Read the model definition and answer for the solid it produces. Units are mm, in the model's axes. A direction names the side the tool comes from. Round coordinates to 2 decimals unless told otherwise and drop trailing zeros. Order: outer loops, then holes, each group sorted by start corner. A loop starts at its lowest first (then second) coordinate and runs counter-clockwise, first axis right, second up. Notation, with made-up numbers: (17.25, 52.25) -> (74.25, 52.25) arc R30 ccw to (74.25, 83.25) -> close; hole circle Ø3 at (50, 9.25). An arc over 180 degrees is marked (long way). Answer as a JSON object with one key per item and string values. Group by question number.
Item 1: For faces 4 (the flat face through (15, 2.4, -2.4)), 5 (the flat face through (93, -12.457, 0)), 6 (the flat face through (52.7, 14.15, -0.07)), determine the directions among +Z, -Z, +X, -X, +Y, -Y from which every point of the face is accessible in a straight line to the end or side of a thin tool.
Item 2: Consider probe 1 along X at (y, z) = (8.5, -3); probe 2 along X at (y, z) = (-10, 5); probe 3 along Z at (x, y) = (85.5, -1). Determine where each line is inside the solid, lowest interval first. Write a range as from..to.
Item 3: The mould has two halves that part along Z. Classify faces 1 (the flat face through (18, 9, 0)), 2 (the cylindrical face through (20.679, 10.657, 9.518)), 3 (the cylindrical face through (94.47, -0.05, -1.25)): pulls with the +Z half, pulls with the -Z half, needs draft (parallel to the pull), parting line crosses it, or undercut.
Item 4: Given P1, Ø0.8, axis at y = 0.5, z = 0, coming from the +X side; P2, Ø4, axis at x = 16, y = 3.5, coming from the -Z side; P3, Ø1.5, axis at x = 93, z = 0, coming from the -Y side, each flat-ended and moving along its own axis, determine where each tip first touches the part or whether it passes through.
Item 5: Section B-B, the plane x = 43 is taken. Write down the section's boundary in (y, z), plus the area to 3 significant figures.
from build123d import *

# Parameters (mm, degrees)
SKETCH_2_OUTSIDE_W       = 55.172
SKETCH_2_OUTSIDE_H       = 55.172
SKETCH_2_OUTSIDE_W_2     = 20
SKETCH_2_OUTSIDE_H_2     = 18
CUT_EXTRUDE_1_DEPTH      = 3
CHAMFER_1_SIZE           = 1
SKETCH_3_R               = 1.5
CUT_EXTRUDE_3_DEPTH      = 3
PATTERN_CIRCULAR_2_COUNT = 4
EXTRUDE_2_DEPTH          = 6
PATTERN_CIRCULAR_3_COUNT = 2


with BuildPart() as part:
    # ｽｹｯﾁ1 → 回転2 (revolve)
    with BuildSketch(Plane(origin=(0, 0, 0), x_dir=(1, 0, 0), z_dir=(0, 1, 0)), mode=Mode.PRIVATE) as revolve_2_sk:
        Polygon((0, 0), (0, 3), (15, 3), (15, 5.5), (15.8, 5.5), (15.8, 7), (16.2, 7), (16.2, 10), (19.2, 10), (19.2, 16), (52.7, 16), (52.7, 14), (90.2, 14), (90.2, 5), (93.2, 5), (93.2, 1.25), (95.7, 1.25), (95.7, 0), align=None)
    revolve(revolve_2_sk.sketch.rotate(Axis((0, 0, 0), (1, 0, 0)), 180), axis=Axis((0, 0, 0), (1, 0, 0)))

    # ｽｹｯﾁ2 outside → ｶｯﾄ - 押し出し1 (cut)
    with BuildSketch(Plane.ZY.offset(-16.2)):
        Rectangle(SKETCH_2_OUTSIDE_W, SKETCH_2_OUTSIDE_H)
        Rectangle(SKETCH_2_OUTSIDE_W_2, SKETCH_2_OUTSIDE_H_2, mode=Mode.SUBTRACT)
    extrude(amount=-CUT_EXTRUDE_1_DEPTH, mode=Mode.SUBTRACT)

    # 面取り1
    chamfer_1_edges = [part.edges().sort_by_distance(p)[0] for p in [
        (19.2, 0, -16),
    ]]
    chamfer(chamfer_1_edges, length=CHAMFER_1_SIZE)

    # ｽｹｯﾁ3 → ｶｯﾄ - 押し出し3 (cut)
    with BuildSketch(Plane.ZY.offset(-19.2)):
        with Locations((-9.192388155, -9.192388155)):
            Circle(SKETCH_3_R)
    cut_extrude_3 = extrude(amount=-CUT_EXTRUDE_3_DEPTH, mode=Mode.SUBTRACT)

    # 円形ﾊﾟﾀｰﾝ2: ｶｯﾄ - 押し出し3 ×4 about axis
    pattern_circular_2_axis = Axis((0, 0, 0), (1, 0, 0))
    for i in range(1, PATTERN_CIRCULAR_2_COUNT):
        add(cut_extrude_3.rotate(pattern_circular_2_axis, i * 360 / PATTERN_CIRCULAR_2_COUNT), mode=Mode.SUBTRACT)

    # ｽｹｯﾁ4 → ﾎﾞｽ - 押し出し2 (add)
    with BuildSketch(Plane(origin=(90.2, 0, 0), x_dir=(0, 0, -1), z_dir=(1, 0, 0))):
        Polygon((0, 12.956973635), (2.5, 12.956973635), (2.5, 12.456973635), (-2.5, 12.456973635), (-2.5, 12.956973635), align=None)
    extrude_2 = extrude(amount=EXTRUDE_2_DEPTH)

    # 円形ﾊﾟﾀｰﾝ3: ﾎﾞｽ - 押し出し2 ×2 about axis
    pattern_circular_3_axis = Axis((0, 0, 0), (1, 0, 0))
    for i in range(1, PATTERN_CIRCULAR_3_COUNT):
        add(extrude_2.rotate(pattern_circular_3_axis, i * 360 / PATTERN_CIRCULAR_3_COUNT))


solid = part.part
Values found:
{
 "1": {"face 4": "-X", "face 5": "+Z, -Z, +X", "face 6": "+X"},
 "2": {"probe 1": "16.2..90.2", "probe 2": "19.2..90.2", "probe 3": "-13.96..13.96"},
 "3": {"face 1": "needs draft", "face 2": "undercut", "face 3": "parting line crosses it"},
 "4": {"P1": "x = 95.7", "P2": "z = -9.89", "P3": "y = -12.96"},
 "5": {"outline": "circle Ø32 at (0, 0)", "area": "804 mm2"}
}
